```python
from build123d import *

# Parameters (mm, degrees)
ESQUISSE1_W                                 = 330
ESQUISSE1_H                                 = 150
ESQUISSE1_R                                 = 4.5
BOSS_EXTRU_1_DEPTH                          = 1.5
FRAISAGE_POUR_VIS_T_TE_FRAIS_E_M31_AT_COUNT = 2
FRAISAGE_POUR_VIS_T_TE_FRAIS_E_M31_AT_PITCH = 17.320508076
FRAISAGE_POUR_VIS_T_TE_FRAIS_E_M31_2_COUNT  = 2
FRAISAGE_POUR_VIS_T_TE_FRAIS_E_M31_2_PITCH  = 17.320508076
CONG_2_R                                    = 10
ESQUISSE4_R                                 = 1.6
ENL_V_MAT_EXTRU_1_DEPTH                     = 205.027571666
CHANFREIN1_SIZE                             = 1.4
FRAISAGE_POUR_VIS_T_TE_FRAIS_E_M32_AT_COUNT = 2
FRAISAGE_POUR_VIS_T_TE_FRAIS_E_M32_AT_PITCH = 20
FRAISAGE_POUR_VIS_T_TE_FRAIS_E_M32_2_COUNT  = 2
FRAISAGE_POUR_VIS_T_TE_FRAIS_E_M32_2_PITCH  = 152.318744743
FRAISAGE_POUR_VIS_T_TE_FRAIS_E_M32_3_COUNT  = 2
FRAISAGE_POUR_VIS_T_TE_FRAIS_E_M32_3_PITCH  = 151
FRAISAGE_POUR_VIS_T_TE_FRAIS_E_M32_4_COUNT  = 2
FRAISAGE_POUR_VIS_T_TE_FRAIS_E_M32_4_PITCH  = 85.158675424
FRAISAGE_POUR_VIS_T_TE_FRAIS_E_M32_5_COUNT  = 2
FRAISAGE_POUR_VIS_T_TE_FRAIS_E_M32_5_PITCH  = 75.3923073
FRAISAGE_POUR_VIS_T_TE_FRAIS_E_M32_6_COUNT  = 2
FRAISAGE_POUR_VIS_T_TE_FRAIS_E_M32_6_PITCH  = 107.447661678
FRAISAGE_POUR_VIS_T_TE_FRAIS_E_M32_7_COUNT  = 2
FRAISAGE_POUR_VIS_T_TE_FRAIS_E_M32_7_PITCH  = 107.056060081
FRAISAGE_POUR_VIS_T_TE_FRAIS_E_M32_8_COUNT  = 2
FRAISAGE_POUR_VIS_T_TE_FRAIS_E_M32_8_PITCH  = 222.766694099
FRAISAGE_POUR_VIS_T_TE_FRAIS_E_M32_9_COUNT  = 2
FRAISAGE_POUR_VIS_T_TE_FRAIS_E_M32_9_PITCH  = 235.416651917
FRAISAGE_POUR_VIS_T_TE_FRAIS_E_M32_10_COUNT = 2
FRAISAGE_POUR_VIS_T_TE_FRAIS_E_M32_10_PITCH = 235.376294473
FRAISAGE_POUR_VIS_T_TE_FRAIS_E_M32_11_COUNT = 2
FRAISAGE_POUR_VIS_T_TE_FRAIS_E_M32_11_PITCH = 244.364481871
FRAISAGE_POUR_VIS_T_TE_FRAIS_E_M32_12_COUNT = 2
FRAISAGE_POUR_VIS_T_TE_FRAIS_E_M32_12_PITCH = 125.906711497
FRAISAGE_POUR_VIS_T_TE_FRAIS_E_M32_13_COUNT = 2
FRAISAGE_POUR_VIS_T_TE_FRAIS_E_M32_13_PITCH = 104.654192463
FRAISAGE_POUR_VIS_T_TE_FRAIS_E_M32_14_COUNT = 2
FRAISAGE_POUR_VIS_T_TE_FRAIS_E_M32_14_PITCH = 44.300112867
FRAISAGE_POUR_VIS_T_TE_FRAIS_E_M32_15_COUNT = 2
FRAISAGE_POUR_VIS_T_TE_FRAIS_E_M32_15_PITCH = 118.501054848
FRAISAGE_POUR_VIS_T_TE_FRAIS_E_M32_16_COUNT = 2
FRAISAGE_POUR_VIS_T_TE_FRAIS_E_M32_16_PITCH = 161.407868458
FRAISAGE_POUR_VIS_T_TE_FRAIS_E_M32_17_COUNT = 2
FRAISAGE_POUR_VIS_T_TE_FRAIS_E_M32_17_PITCH = 247.290315217
FRAISAGE_POUR_VIS_T_TE_FRAIS_E_M32_18_COUNT = 2
FRAISAGE_POUR_VIS_T_TE_FRAIS_E_M32_18_PITCH = 357.617757774


with BuildPart() as part:
    # Esquisse1 → Boss.-Extru.1 (new body)
    with BuildSketch(Plane(origin=(0, 0, 0), x_dir=(1, 0, 0), z_dir=(0, 1, 0))):
        with Locations((0, 45)):
            Rectangle(ESQUISSE1_W, ESQUISSE1_H)
        with Locations(Location((0, 0, 0), (0, 0, 270))):
            Circle(ESQUISSE1_R, mode=Mode.SUBTRACT)
    extrude(amount=BOSS_EXTRU_1_DEPTH)

    # Esquisse3 → Fraisage pour vis à tête fraisée M31 (revolve, cut)
    with BuildSketch(Plane(origin=(5, 0, -8.660254038), x_dir=(0, 0, -1), z_dir=(1, 0, 0))):
        Polygon((0, 0), (0, 1.5), (1.6, 1.5), (1.6, 1.4), (3, 0), align=None)
    fraisage_pour_vis_t_te_frais_e_m31 = revolve(axis=Axis((5, -6.35, -8.660254038), (0, 1, 0)), mode=Mode.SUBTRACT)

    # Fraisage pour vis à tête fraisée M31 at: Fraisage pour vis à tête fraisée M31 ×2
    with Locations(*[(0, 0, i * FRAISAGE_POUR_VIS_T_TE_FRAIS_E_M31_AT_PITCH) for i in range(1, FRAISAGE_POUR_VIS_T_TE_FRAIS_E_M31_AT_COUNT)]):
        add(fraisage_pour_vis_t_te_frais_e_m31, mode=Mode.SUBTRACT)

    # Fraisage pour vis _ t_te frais_e M31 2: Fraisage pour vis à tête fraisée M31 ×2
    with Locations(*[Vector(-0.8660254037844397, 0, 0.49999999999999806) * (i * FRAISAGE_POUR_VIS_T_TE_FRAIS_E_M31_2_PITCH) for i in range(1, FRAISAGE_POUR_VIS_T_TE_FRAIS_E_M31_2_COUNT)]):
        add(fraisage_pour_vis_t_te_frais_e_m31, mode=Mode.SUBTRACT)

    # Congé2
    cong_2_edges = [part.edges().sort_by_distance(p)[0] for p in [
        (-165, 0.75, -120),
        (165, 0.75, -120),
        (165, 0.75, 30),
        (-165, 0.75, 30),
    ]]
    fillet(cong_2_edges, radius=CONG_2_R)

    # Esquisse4 → Enlèv. mat.-Extru.1 (cut, through all)
    with BuildSketch(Plane(origin=(0, 1.5, 0), x_dir=(1, 0, 0), z_dir=(0, 1, 0))):
        with Locations(Location((-102.23074819, 13.000761956, 0), (0, 0, 270))):
            Circle(ESQUISSE4_R)
        with Locations(Location((-118.1975933, 77.04027989, 0), (0, 0, 270))):
            Circle(ESQUISSE4_R)
        with Locations(Location((15, 72.5, 0), (0, 0, 270))):
            Circle(ESQUISSE4_R)
        with Locations(Location((-7.5, 85.490381057, 0), (0, 0, 270))):
            Circle(ESQUISSE4_R)
        with Locations(Location((-7.5, 59.509618943, 0), (0, 0, 270))):
            Circle(ESQUISSE4_R)
        with Locations(Location((0, 72.5, 0), (0, 0, 270))):
            Circle(ESQUISSE4_R)
    extrude(amount=-ENL_V_MAT_EXTRU_1_DEPTH, mode=Mode.SUBTRACT)

    # Chanfrein1
    chanfrein1_edges = [part.edges().sort_by_distance(p)[0] for p in [
        (-102.23074819, 0, -14.600761956),
        (-7.5, 0, -61.109618943),
        (15, 0, -74.1),
        (-7.5, 0, -87.090381057),
        (-118.1975933, 0, -78.64027989),
    ]]
    chamfer(chanfrein1_edges, length=CHANFREIN1_SIZE)

    # Esquisse6 → Fraisage pour vis à tête fraisée M32 (revolve, cut)
    with BuildSketch(Plane(origin=(75.5, 0, -3.5), x_dir=(0, 0, -1), z_dir=(1, 0, 0))):
        Polygon((0, 0), (0, 1.5), (1.7, 1.5), (1.7, 1.45), (3.15, 0), align=None)
    fraisage_pour_vis_t_te_frais_e_m32 = revolve(axis=Axis((75.5, -6.35, -3.5), (0, 1, 0)), mode=Mode.SUBTRACT)

    # Fraisage pour vis à tête fraisée M32 at: Fraisage pour vis à tête fraisée M32 ×2
    with Locations(*[(0, 0, i * FRAISAGE_POUR_VIS_T_TE_FRAIS_E_M32_AT_PITCH) for i in range(1, FRAISAGE_POUR_VIS_T_TE_FRAIS_E_M32_AT_COUNT)]):
        add(fraisage_pour_vis_t_te_frais_e_m32, mode=Mode.SUBTRACT)

    # Fraisage pour vis _ t_te frais_e M32 2: Fraisage pour vis à tête fraisée M32 ×2
    with Locations(*[Vector(-0.9913422031874387, 0, 0.1313036030711839) * (i * FRAISAGE_POUR_VIS_T_TE_FRAIS_E_M32_2_PITCH) for i in range(1, FRAISAGE_POUR_VIS_T_TE_FRAIS_E_M32_2_COUNT)]):
        add(fraisage_pour_vis_t_te_frais_e_m32, mode=Mode.SUBTRACT)

    # Fraisage pour vis _ t_te frais_e M32 3: Fraisage pour vis à tête fraisée M32 ×2
    with Locations(*[(-i * FRAISAGE_POUR_VIS_T_TE_FRAIS_E_M32_3_PITCH, 0, 0) for i in range(1, FRAISAGE_POUR_VIS_T_TE_FRAIS_E_M32_3_COUNT)]):
        add(fraisage_pour_vis_t_te_frais_e_m32, mode=Mode.SUBTRACT)

    # Fraisage pour vis _ t_te frais_e M32 4: Fraisage pour vis à tête fraisée M32 ×2
    with Locations(*[Vector(0.9863939238321435, 0, 0.1643989873053589) * (i * FRAISAGE_POUR_VIS_T_TE_FRAIS_E_M32_4_PITCH) for i in range(1, FRAISAGE_POUR_VIS_T_TE_FRAIS_E_M32_4_COUNT)]):
        add(fraisage_pour_vis_t_te_frais_e_m32, mode=Mode.SUBTRACT)

    # Fraisage pour vis _ t_te frais_e M32 5: Fraisage pour vis à tête fraisée M32 ×2
    with Locations(*[Vector(0.9284766908852593, 0, 0.3713906763541037) * (i * FRAISAGE_POUR_VIS_T_TE_FRAIS_E_M32_5_PITCH) for i in range(1, FRAISAGE_POUR_VIS_T_TE_FRAIS_E_M32_5_COUNT)]):
        add(fraisage_pour_vis_t_te_frais_e_m32, mode=Mode.SUBTRACT)

    # Fraisage pour vis _ t_te frais_e M32 6: Fraisage pour vis à tête fraisée M32 ×2
    with Locations(*[Vector(0.7817759706301133, 0, -0.6235594051454475) * (i * FRAISAGE_POUR_VIS_T_TE_FRAIS_E_M32_6_PITCH) for i in range(1, FRAISAGE_POUR_VIS_T_TE_FRAIS_E_M32_6_COUNT)]):
        add(fraisage_pour_vis_t_te_frais_e_m32, mode=Mode.SUBTRACT)

    # Fraisage pour vis _ t_te frais_e M32 7: Fraisage pour vis à tête fraisée M32 ×2
    with Locations(*[Vector(0.6538630316419344, 0, -0.7566129366142366) * (i * FRAISAGE_POUR_VIS_T_TE_FRAIS_E_M32_7_PITCH) for i in range(1, FRAISAGE_POUR_VIS_T_TE_FRAIS_E_M32_7_COUNT)]):
        add(fraisage_pour_vis_t_te_frais_e_m32, mode=Mode.SUBTRACT)

    # Fraisage pour vis _ t_te frais_e M32 8: Fraisage pour vis à tête fraisée M32 ×2
    with Locations(*[Vector(-0.9920693077275461, 0, 0.12569203898810538) * (i * FRAISAGE_POUR_VIS_T_TE_FRAIS_E_M32_8_PITCH) for i in range(1, FRAISAGE_POUR_VIS_T_TE_FRAIS_E_M32_8_COUNT)]):
        add(fraisage_pour_vis_t_te_frais_e_m32, mode=Mode.SUBTRACT)

    # Fraisage pour vis _ t_te frais_e M32 9: Fraisage pour vis à tête fraisée M32 ×2
    with Locations(*[Vector(-0.9982301510364278, 0, 0.05946903027451117) * (i * FRAISAGE_POUR_VIS_T_TE_FRAIS_E_M32_9_PITCH) for i in range(1, FRAISAGE_POUR_VIS_T_TE_FRAIS_E_M32_9_COUNT)]):
        add(fraisage_pour_vis_t_te_frais_e_m32, mode=Mode.SUBTRACT)

    # Fraisage pour vis _ t_te frais_e M32 10: Fraisage pour vis à tête fraisée M32 ×2
    with Locations(*[Vector(-0.9389220800441849, 0, -0.344129812142891) * (i * FRAISAGE_POUR_VIS_T_TE_FRAIS_E_M32_10_PITCH) for i in range(1, FRAISAGE_POUR_VIS_T_TE_FRAIS_E_M32_10_COUNT)]):
        add(fraisage_pour_vis_t_te_frais_e_m32, mode=Mode.SUBTRACT)

    # Fraisage pour vis _ t_te frais_e M32 11: Fraisage pour vis à tête fraisée M32 ×2
    with Locations(*[Vector(-0.9616782201769339, 0, -0.27418059894406194) * (i * FRAISAGE_POUR_VIS_T_TE_FRAIS_E_M32_11_PITCH) for i in range(1, FRAISAGE_POUR_VIS_T_TE_FRAIS_E_M32_11_COUNT)]):
        add(fraisage_pour_vis_t_te_frais_e_m32, mode=Mode.SUBTRACT)

    # Fraisage pour vis _ t_te frais_e M32 12: Fraisage pour vis à tête fraisée M32 ×2
    with Locations(*[Vector(0.5917079329146707, 0, -0.8061524186689808) * (i * FRAISAGE_POUR_VIS_T_TE_FRAIS_E_M32_12_PITCH) for i in range(1, FRAISAGE_POUR_VIS_T_TE_FRAIS_E_M32_12_COUNT)]):
        add(fraisage_pour_vis_t_te_frais_e_m32, mode=Mode.SUBTRACT)

    # Fraisage pour vis _ t_te frais_e M32 13: Fraisage pour vis à tête fraisée M32 ×2
    with Locations(*[Vector(-0.2436596126725799, 0, -0.9698608112261514) * (i * FRAISAGE_POUR_VIS_T_TE_FRAIS_E_M32_13_PITCH) for i in range(1, FRAISAGE_POUR_VIS_T_TE_FRAIS_E_M32_13_COUNT)]):
        add(fraisage_pour_vis_t_te_frais_e_m32, mode=Mode.SUBTRACT)

    # Fraisage pour vis _ t_te frais_e M32 14: Fraisage pour vis à tête fraisée M32 ×2
    with Locations(*[Vector(-0.8013523601360025, 0, -0.5981926068620863) * (i * FRAISAGE_POUR_VIS_T_TE_FRAIS_E_M32_14_PITCH) for i in range(1, FRAISAGE_POUR_VIS_T_TE_FRAIS_E_M32_14_COUNT)]):
        add(fraisage_pour_vis_t_te_frais_e_m32, mode=Mode.SUBTRACT)

    # Fraisage pour vis _ t_te frais_e M32 15: Fraisage pour vis à tête fraisée M32 ×2
    with Locations(*[Vector(-0.9746748680719794, 0, -0.223626701332532) * (i * FRAISAGE_POUR_VIS_T_TE_FRAIS_E_M32_15_PITCH) for i in range(1, FRAISAGE_POUR_VIS_T_TE_FRAIS_E_M32_15_COUNT)]):
        add(fraisage_pour_vis_t_te_frais_e_m32, mode=Mode.SUBTRACT)

    # Fraisage pour vis _ t_te frais_e M32 16: Fraisage pour vis à tête fraisée M32 ×2
    with Locations(*[Vector(-0.777533345798627, 0, -0.6288417099486903) * (i * FRAISAGE_POUR_VIS_T_TE_FRAIS_E_M32_16_PITCH) for i in range(1, FRAISAGE_POUR_VIS_T_TE_FRAIS_E_M32_16_COUNT)]):
        add(fraisage_pour_vis_t_te_frais_e_m32, mode=Mode.SUBTRACT)

    # Fraisage pour vis _ t_te frais_e M32 17: Fraisage pour vis à tête fraisée M32 ×2
    with Locations(*[Vector(-0.9118836692102092, 0, -0.41044874689506083) * (i * FRAISAGE_POUR_VIS_T_TE_FRAIS_E_M32_17_PITCH) for i in range(1, FRAISAGE_POUR_VIS_T_TE_FRAIS_E_M32_17_COUNT)]):
        add(fraisage_pour_vis_t_te_frais_e_m32, mode=Mode.SUBTRACT)

    # Fraisage pour vis _ t_te frais_e M32 18: Fraisage pour vis à tête fraisée M32 ×2
    with Locations(*[Vector(-0.9699587949702458, 0, 0.24326926657485654) * (i * FRAISAGE_POUR_VIS_T_TE_FRAIS_E_M32_18_PITCH) for i in range(1, FRAISAGE_POUR_VIS_T_TE_FRAIS_E_M32_18_COUNT)]):
        add(fraisage_pour_vis_t_te_frais_e_m32, mode=Mode.SUBTRACT)


solid = part.part
```
The listing builds one solid part. Answer for the finished solid, in the listing's coordinates (mm). Coordinates: 2 decimals unless noted, no trailing zeros. One line per item, written item: value.
1) Find section A-A (y = 0.3). Count the separate pieces of the cut face and the enclosed holes in it, and give its area (3 significant figures).
Geometry check:
separate pieces: 1
enclosed holes: 28
area: 48,700 mm2
2) Consider line 1 along X through (y, z) = (0.7, -72.5); line 2 along Z through (x, y) = (143.5, 0.85); line 3 along X through (y, z) = (0.7, -3.5). Determine where each line is inside the solid, lowest interval first. Write a range as from..to.
Geometry check:
line 1: x = -165..-160.92, -158.08..-1.6, 1.6..12.7, 17.3..158.08, 160.92..165
line 2: z = -120..-85.64, -83.36..23.36, 25.64..30
line 3: x = -165..-77.95, -73.05..-2.83, 2.83..73.05, 77.95..165
3) For a pull along Z with two mould halves and no side action, classify faces 1 (the cylindrical face through (1.352, 0.74, 4.292)), 2 (the flat face through (-2, 1.5, -46)) as pulls with the +Z half, pulls with the -Z half, needs draft (parallel to the pull), parting line crosses it, or undercut.
Geometry check:
face 1: undercut
face 2: needs draft
4) Each of these flat-tipped pins is pushed along its axis until it touches: pin 1 Ø4.5 at (x, z) = (150, -105) entering from +Y; pin 2 Ø4.5 at (x, z) = (145.5, -84.5) entering from -Y; pin 3 Ø5.5 at (x, z) = (75.5, -3.5) entering from -Y; pin 4 Ø2 at (x, z) = (-40, -30) entering from -Y. Where does it stop, or does it pass through?
Geometry check:
pin 1: stops at y = 1.5
pin 2: stops at y = 0.9
pin 3: stops at y = 0.4
pin 4: passes through
